Could you check a few things on this drawing? It's one solid part, dimensions in mm from its lowest x, y, z. Give positions to 0.01 mm unless a question says otherwise; leave off trailing zeros. Loops run counter-clockwise (first coordinate to the right, second up) from the corner with the lowest first, then second, coordinate; pieces in that order, holes last. Notation, with made-up numbers: (28, 18) -> (47, 18) arc R18 ccw to (47, 40) -> close; hole circle Ø11 at (-31, -17). An arc over 180 degrees is marked (long way). Use CSV: the item, a comma, the result in double quotes.
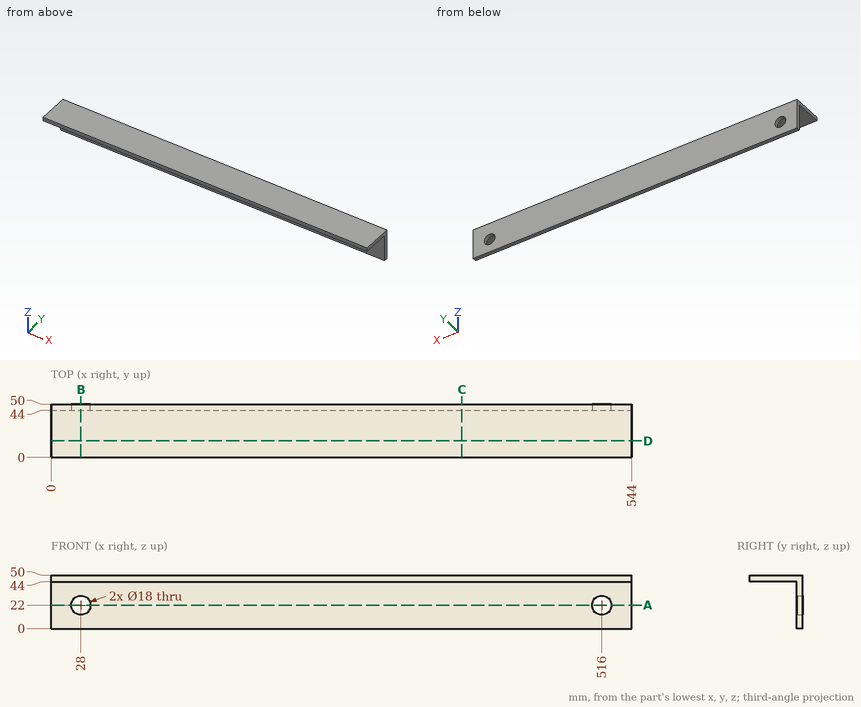
(1) If I drill on L1, parallel to Z at x = 28, y = 47; L2, parallel to Y at x = 519.5, z = 34, over which ranges is the centre line in solid material (lowest first)? Write a range as from..to.
Answer sheet:
L1,"z = 0..13, 31..50"
L2,"y = 44..50"
(2) If we section it at C-C, the plane x = 385: Write out the boundary of the cut face in (y, z), then the cut area to 3 significant figures.
Answer sheet:
outline,"(0, 44) -> (44, 44) -> (44, 0) -> (50, 0) -> (50, 50) -> (0, 50) -> close"
area,"564 mm2"
(3) If we section it at D-D, the plane y = 15.5: Write out the boundary of the cut face in (x, z).
Answer sheet:
outline,"(0, 44) -> (544, 44) -> (544, 50) -> (0, 50) -> close"
(4) If we section it at A-A, the plane z = 22: Write out the boundary of the cut face in (x, y), then the cut area to 3 significant figures.
Answer sheet:
outline,"(0, 44) -> (19, 44) -> (19, 50) -> (0, 50) -> close; (37, 44) -> (507, 44) -> (507, 50) -> (37, 50) -> close; (525, 44) -> (544, 44) -> (544, 50) -> (525, 50) -> close"
area,"3,050 mm2"
(5) If we section it at B-B, the plane x = 28: Write out the boundary of the cut face in (y, z).
Answer sheet:
outline,"(0, 44) -> (44, 44) -> (44, 31) -> (50, 31) -> (50, 50) -> (0, 50) -> close; (44, 0) -> (50, 0) -> (50, 13) -> (44, 13) -> close"
(6) Will this pin go through, and if not, where does the flat tip stop? pin 1 Ø13 at (x, z) = (399, 21.5) entering from -Y.
Answer sheet:
pin 1,"stops at y = 44"
